Could you check a few things on this model? Use its own coordinates, in mm. Face numbers are marked on the shaded views. Give positions to 0.01 mm unless a question says otherwise; leave off trailing zeros. Write each loop counter-clockwise with the first axis right and the second up, starting at its lowest first coordinate (ties: lowest second). Pieces come first, ordered by that corner, then holes. Notation, with made-up numbers: M 38,57.5 L 95,57.5 A22 ccw 95,87.5 Z; hole C -21.75,75.5 d7. An arc over 180 degrees is marked long. Use one line per item in the form item = value.
from build123d import *

# Parameters (mm, degrees)
SKETCH_1_W      = 180
SKETCH_1_H      = 80
EXTRUDE_1_DEPTH = 1.5
SKETCH_2_W      = 152.95364467
SKETCH_2_H      = 2
EXTRUDE_2_DEPTH = 10


with BuildPart() as part:
    # 草图1 → 凸台-拉伸1 (new body)
    with BuildSketch(Plane(origin=(0, 0, 0), x_dir=(1, 0, 0), z_dir=(0, 1, 0))):
        with Locations((0, 0.134932534)):
            Rectangle(SKETCH_1_W, SKETCH_1_H)
        Polygon((37.76, 35), (36.76, 34), (35.76, 35), (36.76, 36), align=None, mode=Mode.SUBTRACT)
        Polygon((-36.76, 34), (-35.76, 35), (-36.76, 36), (-37.76, 35), align=None, mode=Mode.SUBTRACT)
        Polygon((36.76, -36), (37.76, -35), (36.76, -34), (35.76, -35), align=None, mode=Mode.SUBTRACT)
        Polygon((-37.76, -35), (-36.76, -34), (-35.76, -35), (-36.76, -36), align=None, mode=Mode.SUBTRACT)
        Polygon((81, -35), (80, -36), (79, -35), (80, -34), align=None, mode=Mode.SUBTRACT)
        Polygon((80, 36), (79, 35), (80, 34), (81, 35), align=None, mode=Mode.SUBTRACT)
    extrude(amount=EXTRUDE_1_DEPTH)

    # 草图2 → 凸台-拉伸2 (add)
    with BuildSketch(Plane(origin=(0, 1.5, 0), x_dir=(1, 0, 0), z_dir=(0, 1, 0))):
        with Locations((0, 28)):
            Rectangle(SKETCH_2_W, SKETCH_2_H)
        with Locations((0, -28)):
            Rectangle(SKETCH_2_W, SKETCH_2_H)
    extrude(amount=EXTRUDE_2_DEPTH)


solid = part.part
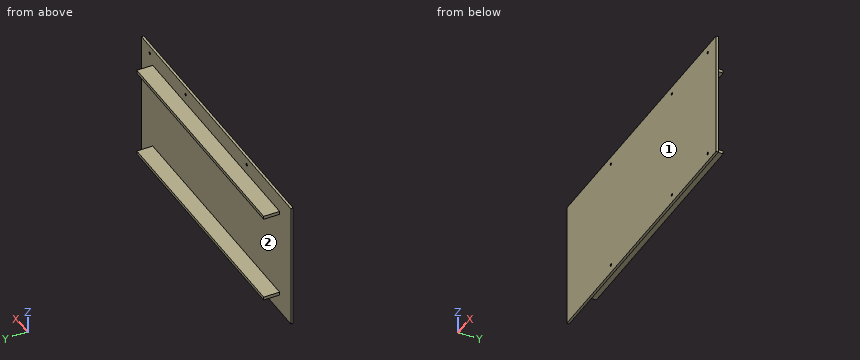
1) I want a section at C-C, the plane z = -16. Please give me the cut outline in (x, y), plus the area to 3 significant figures.
Checked values:
outline = M -90,0 L 90,0 L 90,1.5 L -90,1.5 Z
area = 270 mm2
2) For pin 1 Ø3 at (x, y) = (15, 8.5) entering from +Z; pin 2 Ø1 at (y, z) = (9, -27.5) entering from -X; pin 3 Ø12 at (x, z) = (-71.5, 3) entering from +Y, each with a flat end and sliding along its axis, tell me the tip position at first contact or that it passes through.
Checked values:
pin_1 = 29
pin_2 = -76.48
pin_3 = 1.5
3) Thinking about a two-plate mould opening in Z: for the marked faces 1 and 2, which applies, released by +Z, released by -Z, zero draft, split by the parting line, or undercut?
Checked values:
face_1 = zero draft
face_2 = undercut
4) I want a section at A-A, the plane y = 8.5. Please give me the cut outline in (x, z), plus the area to 3 significant figures.
Checked values:
outline = M -76.48,-29 L 76.48,-29 L 76.48,-27 L -76.48,-27 Z; M -76.48,27 L 76.48,27 L 76.48,29 L -76.48,29 Z
area = 612 mm2
5) I want a section at B-B, the plane x = -9. Please give me the cut outline in (y, z), plus the area to 3 significant figures.
Checked values:
outline = M 0,-40.13 L 1.5,-40.13 L 1.5,-29 L 11.5,-29 L 11.5,-27 L 1.5,-27 L 1.5,27 L 11.5,27 L 11.5,29 L 1.5,29 L 1.5,39.87 L 0,39.87 Z
area = 160 mm2
6) If I drill on L1, parallel to Z at x = 59, y = 10.75; L2, parallel to Y at x = 25, z = -34.5, over which ranges is the centre line in solid material (lowest first)?
Checked values:
L1 = -29 to -27, 27 to 29
L2 = 0 to 1.5
